Design review of the part built by this model. Coordinates are the model's own, in mm. Give positions to 0.01 mm unless a question says otherwise; leave off trailing zeros. Write each loop counter-clockwise with the first axis right and the second up, starting at its lowest first coordinate (ties: lowest second). Pieces come first, ordered by that corner, then holes. Notation, with made-up numbers: M 19,40 L 42,40 A35 ccw 42,75 Z; hole C 24.25,-16.5 d9. An arc over 180 degrees is marked long. Use one line per item in the form item = value. Start each with the question number.
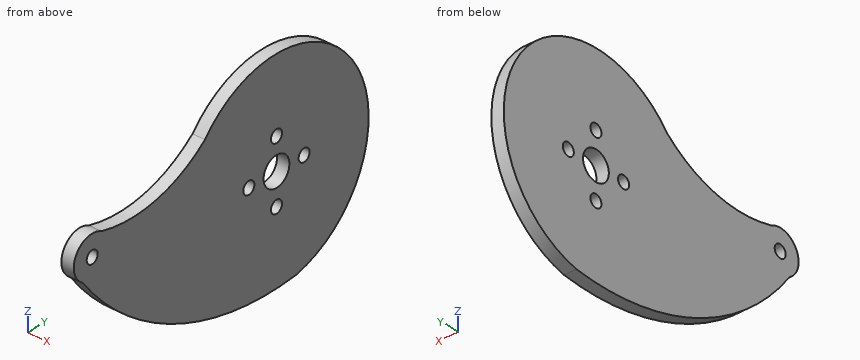
from build123d import *

# Parameters (mm, degrees)
CROQUIS1_R              = 3.5
CROQUIS1_R_2            = 1.5
SALIENTE_EXTRUIR1_DEPTH = 3


with BuildPart() as part:
    # Croquis1 → Saliente-Extruir1 (new body)
    with BuildSketch(Plane(origin=(0, 0, 0), x_dir=(0, 0, -1), z_dir=(1, 0, 0))):
        with BuildLine():
            ThreePointArc((24.429451457, 5.310546254), (-13.102683121, 21.291305621), (-15.74927408, -19.415467184))
            ThreePointArc((-15.74927408, -19.415467184), (-9.07160693, -32.67265708), (-9.338328875, -47.514260157))
            ThreePointArc((-9.338328875, -47.514260157), (-7.527733898, -54.313995983), (-0.71074339, -52.569489781))
            ThreePointArc((-0.71074339, -52.569489781), (19.815359954, -27.085163099), (24.429451457, 5.310546254))
        make_face()
        Circle(CROQUIS1_R, mode=Mode.SUBTRACT)
        with Locations((-5, -50)):
            Circle(CROQUIS1_R_2, mode=Mode.SUBTRACT)
        with Locations((-7.5, 0)):
            Circle(CROQUIS1_R_2, mode=Mode.SUBTRACT)
        with Locations((0, 7.5)):
            Circle(CROQUIS1_R_2, mode=Mode.SUBTRACT)
        with Locations((7.5, 0)):
            Circle(CROQUIS1_R_2, mode=Mode.SUBTRACT)
        with Locations((0, -7.5)):
            Circle(CROQUIS1_R_2, mode=Mode.SUBTRACT)
    extrude(amount=SALIENTE_EXTRUIR1_DEPTH)


solid = part.part
1. We need section D-D (y = 0). State the section outline as (x, z) points, and give its area (3 significant figures).
2. We need section B-B (y = -50). State the section outline as (x, z) points, and give its area (3 significant figures).
3. Clearance check with flat-ended pins moving along their axes: pin 1 Ø6 at (y, z) = (-34, -18.5) entering from -X; pin 2 Ø1.5 at (x, z) = (0.5, 14.5) entering from -Y; pin 3 Ø1 at (x, z) = (1.5, 11.5) entering from -Y; pin 4 Ø4 at (y, z) = (0, 0) entering from +X. State where each tip first meets the part, or that it passes through.
4. To check wall thickness, follow L1, parallel to Y at x = 1.8, z = 0; L2, parallel to Y at x = 1.35, z = -0.5 (3 decimals); L3, parallel to Y at x = 1.95, z = 5. State the ranges of each line that lie inside material, in increasing order.
5. We need section A-A (z = -7.5). State the section outline as (x, y) points.
6. We need section C-C (x = 1.1). State the section outline as (y, z) points.
Answer block:
q1.outline = M 0,-24.87 L 3,-24.87 L 3,-9 L 0,-9 Z; M 0,-6 L 3,-6 L 3,-3.5 L 0,-3.5 Z; M 0,3.5 L 3,3.5 L 3,6 L 0,6 Z; M 0,9 L 3,9 L 3,25 L 0,25 Z
q1.area = 111 mm^2
q2.outline = M 0,-2.61 L 3,-2.61 L 3,3.5 L 0,3.5 Z; M 0,6.5 L 3,6.5 L 3,10 L 0,10 Z
q2.area = 28.8 mm^2
q3.pin_1 = 0
q3.pin_2 = -22.01
q3.pin_3 = -26.91
q3.pin_4 = through
q4.L1 = -52.05 to -9, -6 to -3.5, 3.5 to 6, 9 to 25
q4.L2 = -51.674 to -8.914, -6.086 to -3.464, 3.464 to 6.086, 8.914 to 24.995
q4.L3 = -55 to -51.5, -48.5 to 24.49
q5.outline = M 0,-45.48 L 3,-45.48 L 3,-1.5 L 0,-1.5 Z; M 0,1.5 L 3,1.5 L 3,23.85 L 0,23.85 Z
q6.outline = M -52.57,0.71 A61.72 ccw 5.31,-24.43 A25 ccw long -19.42,15.75 A30.93 cw -47.51,9.34 A5 ccw Z; hole C -50,5 d3; hole C -7.5,0 d3; hole C 0,0 d7; hole C 0,-7.5 d3; hole C 0,7.5 d3; hole C 7.5,0 d3
